Autodesk Inventor part; units mm, degrees
ref_plane "Work Plane1" through (0, 25.4, 0) normal (0, 1, 0) x (-1, 0, 0)
ref_plane "YZ Plane" through (0, 0, 0) normal (1, 0, 0) x (0, 1, 0)
ref_plane "XY Plane" through (0, 0, 0) normal (0, 0, 1) x (1, 0, 0)
sketch "Sketch1" plane through (0, 0, 0) normal (0, 1, 0) x (-1, 0, 0)
  line L0 (0, 0) -> (69.85, 0)
  line L1 (69.85, 0) -> (69.85, -304.8)
  line L2 (69.85, -304.8) -> (0, -304.8)
  line L3 (0, -304.8) -> (0, 0)
  dimension "d0" = 69.85
  dimension "d1" = 304.8
ref_plane "Work Plane1" through (0, 25.4, 0) normal (0, 1, 0) x (-1, 0, 0)
sketch "Sketch2" plane through (0, 25.4, 0) normal (0, 1, 0) x (-1, 0, 0)
  line L0 (0, 0) -> (69.85, 0)
  line L1 (69.85, 0) -> (69.85, -304.8)
  line L2 (69.85, -304.8) -> (0, -304.8)
  line L3 (0, -304.8) -> (0, 0)
  line L4 (63.5, -298.45) -> (63.5, -6.35)
  line L5 (63.5, -6.35) -> (6.35, -6.35)
  line L6 (6.35, -6.35) -> (6.35, -298.45)
  line L7 (6.35, -298.45) -> (63.5, -298.45)
  dimension "d3" = 6.35
loft "Loft1" add profiles "Sketch1", "Sketch2" contours all / L7 L6 L5 L4
sketch "Sketch3" plane through (-63.5, 25.4, -6.35) normal (0, 1, 0) x (1, 0, 0)
  line L0 (57.15, 0) -> (0, 0)
  line L1 (57.15, 292.1) -> (57.15, 0)
  line L2 (0, 292.1) -> (57.15, 292.1)
  line L3 (0, 0) -> (0, 292.1)
  line L4 (50.8, 6.35) -> (6.35, 6.35)
  line L5 (6.35, 285.75) -> (50.8, 285.75)
  line L6 (50.8, 285.75) -> (50.8, 6.35)
  line L7 (6.35, 12.7) -> (44.45, 12.7)
  line L8 (44.45, 12.7) -> (44.45, 279.4)
  line L9 (44.45, 279.4) -> (6.35, 279.4)
  line L10 (6.35, 6.35) -> (6.35, 12.7)
  line L11 (6.35, 279.4) -> (6.35, 285.75)
  circle A0 centre (12.7, 50.8) radius 6.35
  circle A1 centre (12.7, 88.9) radius 6.35
  circle A2 centre (12.7, 127) radius 6.35
  circle A3 centre (12.7, 165.1) radius 6.35
  circle A4 centre (12.7, 203.2) radius 6.35
  circle A5 centre (12.7, 241.3) radius 6.35
  point P0 (63.5, -6.35)
  dimension "d8" = 6.35
  dimension "d9" = 12.7
  dimension "d10" = 12.7
  dimension "d11" = 12.7
  dimension "d12" = 12.7
  dimension "d13" = 6.35
  dimension "d14" = 38.1
  dimension "d17" = 38.1
extrude "Extrusion1" add sketch "Sketch3" along normal blind 38.1 contours L4 L10 L7 L8 L9 L11 L5 L6 | A0 | A1 | A2 | A3 | A4 | A5
sketch "Sketch4" plane through (-63.5, 63.5, -6.35) normal (0, 1, 0) x (1, 0, 0)
  line L0 (6.35, 6.35) -> (50.8, 6.35)
  line L1 (50.8, 6.35) -> (50.8, 285.75)
  line L2 (50.8, 285.75) -> (6.35, 285.75)
  line L3 (6.35, 285.75) -> (6.35, 6.35)
  point P0 (63.5, -6.35)
extrude "Extrusion2" add sketch "Sketch4" along normal blind 25.4
properties part number "Side2"
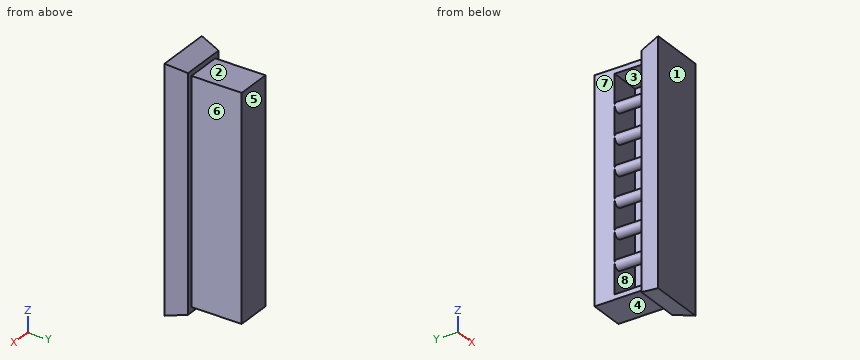
Verification items for the finished model (mm, model axes). Face numbers are marked on the shaded views. A direction names the side the tool comes from. Give positions to 0.01 mm unless a question says otherwise; leave off trailing zeros. Loops run counter-clockwise (first coordinate to the right, second up) from the corner with the lowest first, then second, coordinate; pieces in that order, holes last.
1. Go/stop test with flat-tipped pins: P1, Ø4, axis at x = -56.5, y = 68, coming from the +Z side; P2, Ø6, axis at x = -28.5, y = 20, coming from the -Z side; P3, Ø19, axis at x = -36.5, y = 35.5, coming from the -Z side. Record where each tip stops, or that it passes through.
Derived:
P1: stops at z = -12.7
P2: stops at z = -300.55
P3: stops at z = -292.1
2. Material ranges on probe 1 along Y at (x, z) = (-24.5, -280); probe 2 along Z at (x, y) = (-40, 40.5); probe 3 along Y at (x, z) = (-11.5, -32.5), recorded low to high.
Derived:
probe 1: y = 0 to 25.4, 63.5 to 88.9
probe 2: z = -292.1 to -285.75, -19.05 to -12.7
probe 3: y = 0 to 25.4
3. Cross-section at C-C on y = 75. Record the cut outline in (x, z), and give its area (3 significant figures).
Derived:
outline: (-57.15, -292.1) - (-12.7, -292.1) - (-12.7, -12.7) - (-57.15, -12.7) - close
area: 12,400 mm2
4. Cross-section at A-A on y = 37. Record the cut outline in (x, z).
Derived:
outline: (-57.15, -292.1) - (-12.7, -292.1) - (-12.7, -12.7) - (-57.15, -12.7) - (-57.15, -19.05) - (-19.05, -19.05) - (-19.05, -285.75) - (-57.15, -285.75) - close; circle Ø12.7 at (-50.8, -247.65); circle Ø12.7 at (-50.8, -209.55); circle Ø12.7 at (-50.8, -171.45); circle Ø12.7 at (-50.8, -133.35); circle Ø12.7 at (-50.8, -95.25); circle Ø12.7 at (-50.8, -57.15)
5. Cross-section at B-B on x = -50.8. Count the separate pieces of the cut face and the enclosed holes in it, and give its area (3 significant figures).
Derived:
separate pieces: 1
enclosed holes: 7
area: 18,100 mm2
6. Tool access check on the marked faces 4, 5, 6, 7 and 8. Record the directions out of +Z, -Z, +X, -X, +Y, -Y that give a thin tool (end or side, any length) a straight path to the whole face; none if there is none.
Derived:
face 4: -Z, +X, -X, +Y
face 5: +Z, -Z, +X, -X, +Y
face 6: +Z, -Z, +X, +Y
face 7: +Z, -Z, -X, +Y
face 8: none
7. Release check for a two-part mould opening along Y. For the marked faces 1, 2 and 3 record: +Y half, -Y half, draft (parallel to the pull), parting line (faces both ways), or undercut.
Derived:
face 1: -Y half
face 2: draft
face 3: undercut
